Source: CAD feature listing. Evaluate the final solid. Frame: model axes, mm. Face numbers are marked on the shaded views. A direction names the side the tool comes from. Give positions to 0.01 mm unless a question says otherwise; leave off trailing zeros. Order: outer loops, then holes, each group sorted by start corner. A loop starts at its lowest first (then second) coordinate and runs counter-clockwise, first axis right, second up.
1) Draft query along Y for the marked faces 1, 2, 3 and 4. Return one class per face: released by +Y, released by -Y, zero draft, split by the parting line, or undercut.
2) Section A-A, the plane x = 7. Return loops of the section in (y, z), plus the area to 3 significant figures.
3) Access query for the marked faces 5 and 6. Directions: +Z, -Z, +X, -X, +Y, -Y. A direction counts if a zero-diameter tool reaches every point of the face in a straight line with its end or side. Return the directions, or none.
4) Section B-B, the plane z = 10. Return loops of the section in (x, y).
5) First-contact query: P1, Ø8, axis at y = 7.5, z = 4.5, coming from the +X side. Flat tip, straight axial feed; report the tip coordinate or a pass-through.
6) Material intervals for line 1 (Z direction, x = -1.4, y = 7); line 2 (X direction, y = 6.5, z = 13), sorted ascending.
7) Section D-D, the plane z = 8. Return loops of the section in (x, y).
```python
from build123d import *

# Parameters (mm, degrees)
BOSS_EXTRUDE1_DEPTH = 16
CUT_EXTRUDE1_REACH  = 32.741
SKETCH2_R           = 2.5
CUT_EXTRUDE2_REACH  = 32.741
SKETCH3_R           = 2.5


with BuildPart() as part:
    # Sketch1 → Boss-Extrude1 (new body)
    with BuildSketch(Plane.XY):
        Polygon((0, 0), (0, 17), (-3, 17), (-3, -3), (17, -3), (17, 0), align=None)
    extrude(amount=BOSS_EXTRUDE1_DEPTH)

    # Sketch2 → Cut-Extrude1 (cut, up to next)
    with BuildSketch(Plane.ZY.offset(3), mode=Mode.PRIVATE) as cut_extrude1_sk1:
        with Locations(Location((8, 7, 0), (0, 0, 270))):
            Circle(SKETCH2_R)
    cut_extrude1_tool1 = extrude(cut_extrude1_sk1.sketch, amount=-CUT_EXTRUDE1_REACH, mode=Mode.PRIVATE) & part.part
    add(cut_extrude1_tool1.solids().sort_by_distance((-3, 7, 8))[0], mode=Mode.SUBTRACT)

    # Sketch3 → Cut-Extrude2 (cut, up to next)
    with BuildSketch(Plane.XZ.offset(3), mode=Mode.PRIVATE) as cut_extrude2_sk1:
        with Locations((7, 8)):
            Circle(SKETCH3_R)
    cut_extrude2_tool1 = extrude(cut_extrude2_sk1.sketch, amount=-CUT_EXTRUDE2_REACH, mode=Mode.PRIVATE) & part.part
    add(cut_extrude2_tool1.solids().sort_by_distance((7, -3, 8))[0], mode=Mode.SUBTRACT)


solid = part.part
```
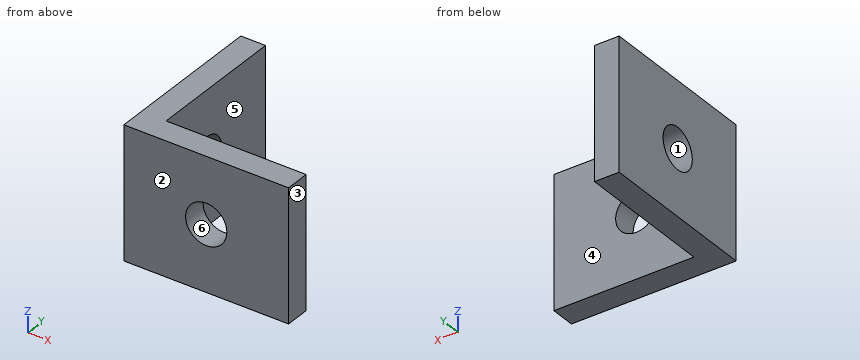
From the geometry:
1. face 1: undercut
1. face 2: released by -Y
1. face 3: zero draft
1. face 4: released by +Y
2. outline: (-3, 0) - (0, 0) - (0, 5.5) - (-3, 5.5) - close; (-3, 10.5) - (0, 10.5) - (0, 16) - (-3, 16) - close
2. area: 33.0 mm2
3. face 5: +Z, -Z, +X, +Y
3. face 6: +Y, -Y
4. outline: (-3, -3) - (5.5, -3) - (5.5, 0) - (0, 0) - (0, 5.5) - (-3, 5.5) - close; (-3, 8.5) - (0, 8.5) - (0, 17) - (-3, 17) - close; (8.5, -3) - (17, -3) - (17, 0) - (8.5, 0) - close
5. P1: stops at x = 0
6. line 1: z = 0 to 5.5, 10.5 to 16
6. line 2: x = -3 to 0
7. outline: (-3, -3) - (4.5, -3) - (4.5, 0) - (0, 0) - (0, 4.5) - (-3, 4.5) - close; (-3, 9.5) - (0, 9.5) - (0, 17) - (-3, 17) - close; (9.5, -3) - (17, -3) - (17, 0) - (9.5, 0) - close
